from build123d import *

# Parameters (mm, degrees)
CROQUIS1_W            = 71
CROQUIS1_H            = 7
EXTRUIR1_DEPTH        = 5.5
CROQUIS2_W            = 65
CROQUIS2_H            = 2.766320183
CORTAR_EXTRUIR1_DEPTH = 7.5
CROQUIS3_W            = 63
CROQUIS3_H            = 2
EXTRUIR2_DEPTH        = 5.5
CROQUIS4_W            = 49.5
CROQUIS4_H            = 2
CROQUIS4_W_2          = 12.5
CORTAR_EXTRUIR2_DEPTH = 2.9
REDONDEO1_R           = 2
CROQUIS5_W            = 15.670728733
CROQUIS5_H            = 1.800640157
CROQUIS5_W_2          = 52.74714617
CORTAR_EXTRUIR3_DEPTH = 2.9


with BuildPart() as part:
    # Croquis1 → Extruir1 (new body)
    with BuildSketch(Plane(origin=(0, 0, 0), x_dir=(1, 0, 0), z_dir=(0, 1, 0))):
        Rectangle(CROQUIS1_W, CROQUIS1_H)
    extrude(amount=EXTRUIR1_DEPTH)

    # Croquis2 → Cortar-Extruir1 (cut)
    with BuildSketch(Plane(origin=(0, 5.5, 0), x_dir=(-1, 0, 0), z_dir=(0, 1, 0))):
        with Locations((0, 3.383160092)):
            Rectangle(CROQUIS2_W, CROQUIS2_H)
    extrude(amount=-CORTAR_EXTRUIR1_DEPTH, mode=Mode.SUBTRACT)

    # Croquis3 → Extruir2 (add)
    with BuildSketch(Plane(origin=(0, 5.5, 0), x_dir=(-1, 0, 0), z_dir=(0, 1, 0))):
        with Locations((0, -4.5)):
            Rectangle(CROQUIS3_W, CROQUIS3_H)
    extrude(amount=-EXTRUIR2_DEPTH)

    # Croquis4 → Cortar-Extruir2 (cut)
    with BuildSketch(Plane(origin=(0, 5.5, 0), x_dir=(-1, 0, 0), z_dir=(0, 1, 0))):
        with Locations((-6.75, -4.5)):
            Rectangle(CROQUIS4_W, CROQUIS4_H)
        with Locations((25.25, -4.5)):
            Rectangle(CROQUIS4_W_2, CROQUIS4_H)
    extrude(amount=-CORTAR_EXTRUIR2_DEPTH, mode=Mode.SUBTRACT)

    # Redondeo1
    redondeo1_edges = [part.edges().sort_by_distance(p)[0] for p in [
        (-18.5, 5.5, -5.5),
    ]]
    fillet(redondeo1_edges, radius=REDONDEO1_R)

    # Croquis5 → Cortar-Extruir3 (cut)
    with BuildSketch(Plane(origin=(0, 0, -3.5), x_dir=(-1, 0, 0), z_dir=(0, 0, -1))):
        with Locations((26.835364367, 4.033789802)):
            Rectangle(CROQUIS5_W, CROQUIS5_H)
        with Locations((-8.373573085, 4.033789802)):
            Rectangle(CROQUIS5_W_2, CROQUIS5_H)
    extrude(amount=-CORTAR_EXTRUIR3_DEPTH, mode=Mode.SUBTRACT)


solid = part.part
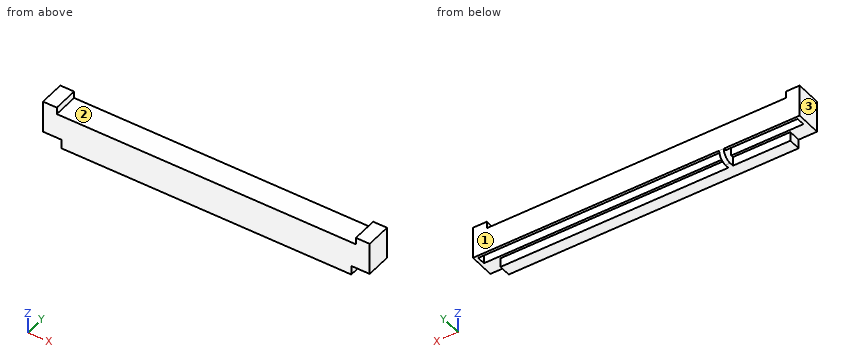
Geometry: final body of the model. Coordinates: model frame, mm. Face numbers are marked on the shaded views. Round coordinates to 2 decimals unless told otherwise and drop trailing zeros. Order: outer loops, then holes, each group sorted by start corner. A loop starts at its lowest first (then second) coordinate and runs counter-clockwise, first axis right, second up. Notation, with made-up numbers: (47.5, 14) - (87.5, 14) arc R11 ccw to (87.5, 30) - close; hole circle Ø7 at (16, 10.25). An arc over 180 degrees is marked (long way). Write each question's results on one line, items separated by ' | '.
Item 1: Section A-A, the plane z = -1.25. Return the cut outline in (x, y).
Completed:
outline: (-35.5, 0) - (35.5, 0) - (35.5, 5.5) - (-35.5, 5.5) - close; hole (-34.67, 3.13) - (-19, 3.13) - (-19, 4.93) - (-34.67, 4.93) - close; hole (-18, 3.13) - (34.75, 3.13) - (34.75, 4.93) - (-18, 4.93) - close
Item 2: First-contact query: pin 1 Ø1.6 at (x, y) = (-14, 2) entering from +Z; pin 2 Ø2 at (x, y) = (9, 4) entering from -Z. Flat tips, straight axial feed; report the tip coordinate or a pass-through.
Completed:
pin 1: z = 2 | pin 2: z = -3.5
Item 3: Section B-B, the plane x = 30.5. Return the cut outline in (y, z), and give its area (3 significant figures).
Completed:
outline: (0, -5.5) - (2.6, -5.5) - (2.6, -3.5) - (3.13, -3.5) - (3.13, -0.6) - (4.93, -0.6) - (4.93, -3.5) - (5.5, -3.5) - (5.5, 2) - (0, 2) - close | area: 30.2 mm^2
Item 4: Material intervals for line 1 along X through (y, z) = (3.85, -1.25); line 2 along Y through (x, z) = (2.5, -3); line 3 along X through (y, z) = (0.5, 2.5), sorted ascending. Write a range as [from, to].
Completed:
line 1: [-35.5, -34.67], [-19, -18], [34.75, 35.5] | line 2: [0, 3.13], [4.93, 5.5] | line 3: [-35.5, -32.5], [32.5, 35.5]
Item 5: Mould query, pull axis X, two halves, no side actions, for the marked faces 1, 2 and 3. Classes: pulls with the +X half, pulls with the -X half, needs draft (parallel to the pull), parting line crosses it, or undercut.
Completed:
face 1: needs draft | face 2: undercut | face 3: pulls with the -X half
Item 6: Section C-C, the plane y = 4.25. Return the cut outline in (x, z), and give its area (3 significant figures).
Completed:
outline: (-35.5, -3.5) - (-34.67, -3.5) - (-34.67, -0.6) - (-19, -0.6) - (-19, -5.35) - (-18, -5.35) - (-18, -0.6) - (34.75, -0.6) - (34.75, -3.5) - (35.5, -3.5) - (35.5, 3.5) - (32.5, 3.5) - (32.5, 2) - (-32.5, 2) - (-32.5, 3.5) - (-35.5, 3.5) - close | area: 203 mm^2
Item 7: Section D-D, the plane z = -4.25. Return the cut outline in (x, y).
Completed:
outline: (-31.5, 0) - (31.5, 0) - (31.5, 2.6) - (-18, 2.6) - (-18, 5.35) - (-19, 5.35) - (-19, 2.6) - (-31.5, 2.6) - close
